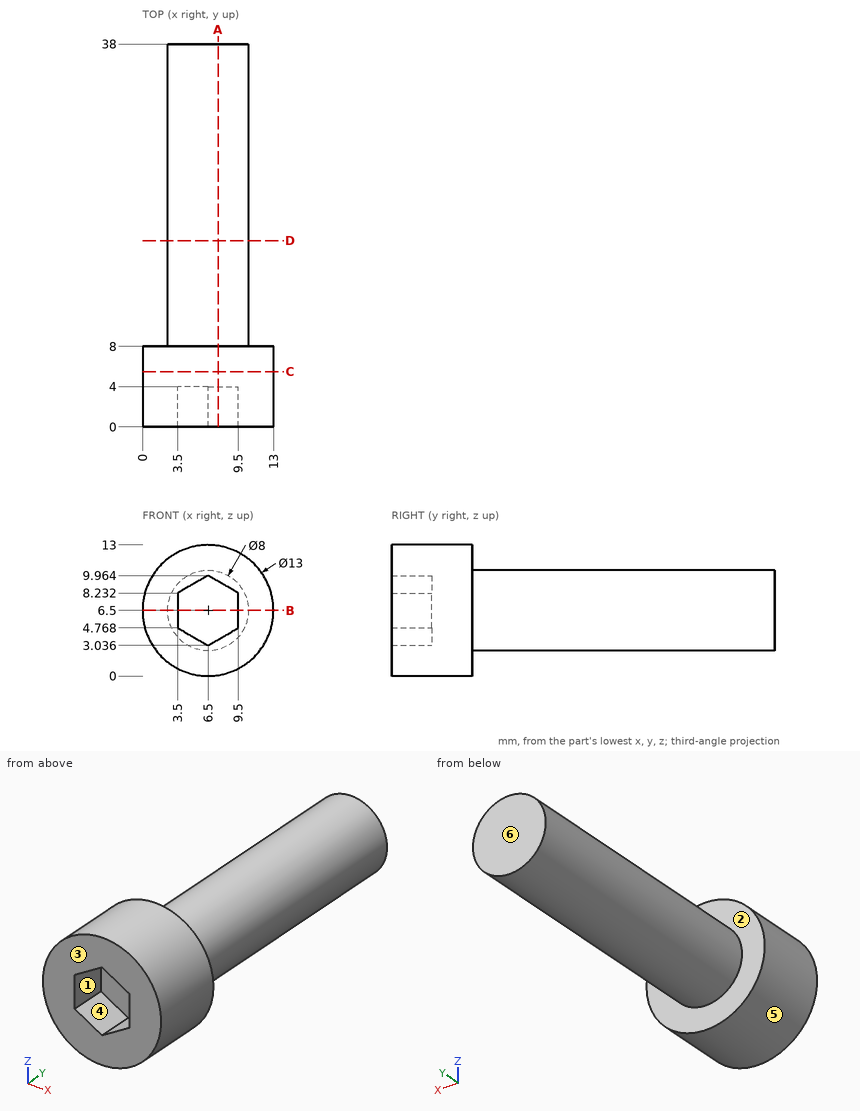
Geometry: see drawing. Coordinates: mm, zero at the bounding-box minimum. A direction names the side the tool comes from. Give positions to 0.01 mm unless a question says otherwise; leave off trailing zeros. Order: outer loops, then holes, each group sorted by start corner. A loop starts at its lowest first (then second) coordinate and runs counter-clockwise, first axis right, second up. Notation, with made-up numbers: (82, 72.25) - (118, 72.25) arc R29 cw to (118, 104.25) - close; hole circle Ø7 at (-27.5, 31.5). An arc over 180 degrees is marked (long way). Use CSV: the item, a comma, the result in double quotes.
1. Section query D-D (y = 18.5). Output: boundary loops of the cut face in (x, z), plus the area to 3 significant figures.
Answers below:
outline,"circle Ø8 at (6.5, 6.5)"
area,"50.3 mm2"
2. Contact query for flat-ended pins moving along their axis: pin 1 (1.7 mm diameter, centred on y = 1, z = 7.5, fed in from -X); pin 2 (3 mm diameter, centred on y = 17.5, z = 3.5, fed in from +X); pin 3 (1 mm diameter, centred on y = 24.5, z = 6.5, fed in from -X). Output: stop coordinate, or through.
Answers below:
pin 1,"x = 0"
pin 2,"x = 10.21"
pin 3,"x = 2.5"
3. Section query A-A (x = 7.5). Output: boundary loops of the cut face in (y, z).
Answers below:
outline,"(0, 0.08) - (8, 0.08) - (8, 2.63) - (38, 2.63) - (38, 10.37) - (8, 10.37) - (8, 12.92) - (0, 12.92) - (0, 9.39) - (4, 9.39) - (4, 3.61) - (0, 3.61) - close"
4. Mould query, pull axis Z, two halves, no side actions, for the marked faces 4, 5 and 6. Classes: +Z half, -Z half, draft (parallel to the pull), parting line (faces both ways), or undercut.
Answers below:
face 4,"undercut"
face 5,"parting line"
face 6,"draft"
5. Section query B-B (z = 6.5). Output: boundary loops of the cut face in (x, y).
Answers below:
outline,"(0, 0) - (3.5, 0) - (3.5, 4) - (9.5, 4) - (9.5, 0) - (13, 0) - (13, 8) - (10.5, 8) - (10.5, 38) - (2.5, 38) - (2.5, 8) - (0, 8) - close"
6. Access query for the marked faces 1, 2 and 3. Directions: +Z, -Z, +X, -X, +Y, -Y. A direction counts if a zero-diameter tool reaches every point of the face in a straight line with its end or side. Return the directions, or none.
Answers below:
face 1,"-Y"
face 2,"+Y"
face 3,"+Z, -Z, +X, -X, -Y"
7. Section query C-C (y = 5.5). Output: boundary loops of the cut face in (x, z), plus the area to 3 significant figures.
Answers below:
outline,"circle Ø13 at (6.5, 6.5)"
area,"133 mm2"
8. Material intervals for line 1 along X through (y, z) = (2.5, 6.25) (3 decimals); line 2 along Y through (x, z) = (10.25, 11.25); line 3 along Y through (x, z) = (4.5, 6.5), sorted ascending. Write a range as from..to.
Answers below:
line 1,"0.005..3.5, 9.5..12.995"
line 2,"0..8"
line 3,"4..38"
